from build123d import *

# Parameters (mm, degrees)
SKETCH1_R           = 5
SKETCH1_R_2         = 1.7
SKETCH1_R_3         = 2
SKETCH1_W           = 142.3736446
SKETCH1_H           = 35.551129401
SKETCH1_H_2         = 35.551129402
BOSS_EXTRUDE1_DEPTH = 2


with BuildPart() as part:
    # Sketch1 → Boss-Extrude1 (new body)
    with BuildSketch(Plane(origin=(0, 0, 0), x_dir=(1, 0, 0), z_dir=(0, 1, 0))):
        Polygon((67.730491212, 150.133829438), (82.230491212, 150.133829438), (85.730491212, 150.133829438), (85.730491212, 100.082700036), (85.730491212, 85.582700036), (85.730491212, 50.031570635), (85.730491212, 32.031570635), (67.730491212, 32.031570635), (62.730491212, 32.031570635), (62.730491212, 35.531570635), (-84.727026002, 35.531570635), (-99.227026002, 35.531570635), (-102.727026002, 35.531570635), (-102.727026002, 85.582700036), (-102.727026002, 92.832700036), (-102.727026002, 98.923608877), (-102.727026002, 100.082700036), (-102.727026002, 153.633829438), (-84.643153388, 153.633829438), (-79.643153388, 153.633829438), (-79.643153388, 153.432122466), (-79.643153388, 150.133829438), align=None)
        with Locations((-91.977026002, 142.883829438)):
            Circle(SKETCH1_R, mode=Mode.SUBTRACT)
        with Locations((74.980491212, 42.781570635)):
            Circle(SKETCH1_R, mode=Mode.SUBTRACT)
        with Locations((-86.427026002, 148.433829438)):
            Circle(SKETCH1_R_2, mode=Mode.SUBTRACT)
        with Locations((-97.527026002, 148.433829438)):
            Circle(SKETCH1_R_2, mode=Mode.SUBTRACT)
        with Locations((-86.427026002, 137.333829438)):
            Circle(SKETCH1_R_2, mode=Mode.SUBTRACT)
        with Locations((-97.527026002, 137.333829438)):
            Circle(SKETCH1_R_2, mode=Mode.SUBTRACT)
        with Locations((69.430491212, 48.331570635)):
            Circle(SKETCH1_R_2, mode=Mode.SUBTRACT)
        with Locations((80.530491212, 48.331570635)):
            Circle(SKETCH1_R_2, mode=Mode.SUBTRACT)
        with Locations((80.530491212, 37.231570635)):
            Circle(SKETCH1_R_2, mode=Mode.SUBTRACT)
        with Locations((69.430491212, 37.231570635)):
            Circle(SKETCH1_R_2, mode=Mode.SUBTRACT)
        with Locations((-54, 92.833829438)):
            Circle(SKETCH1_R_3, mode=Mode.SUBTRACT)
        with Locations((0, 92.833829438)):
            Circle(SKETCH1_R_3, mode=Mode.SUBTRACT)
        with Locations((54, 92.833829438)):
            Circle(SKETCH1_R_3, mode=Mode.SUBTRACT)
        with Locations((-8.456331088, 67.807135336)):
            Rectangle(SKETCH1_W, SKETCH1_H, mode=Mode.SUBTRACT)
        with Locations((-8.456331088, 117.858264737)):
            Rectangle(SKETCH1_W, SKETCH1_H_2, mode=Mode.SUBTRACT)
    extrude(amount=BOSS_EXTRUDE1_DEPTH)


solid = part.part
Here's how the part is built. I have some questions about the finished solid (model axes, mm). Round coordinates to 2 decimals unless told otherwise and drop trailing zeros. Loops run counter-clockwise (first coordinate to the right, second up) from the corner with the lowest first, then second, coordinate; pieces in that order, holes last. Notation, with made-up numbers: M 87.5,57 L 142.5,57 A15 cw 142.5,85 Z; hole C 19.5,27 d9. An arc over 180 degrees is marked long. Write each question's results on one line, items separated by ' | '. Start each with the question number.
(1) Will these pins go through, and if not, where does the flat tip stop? P1, Ø5.5, axis at x = 80.53, z = -37.23, coming from the -Y side; P2, Ø1, axis at x = -58, y = 1, coming from the +Z side.
(2) I want a section at C-C (x = -54). Please give me the cut outline in (y, z).
(3) Thinking about a two-plate mould opening in Z: for faces 1 (the flat face through (-7, 2, -94)), 2 (the cylindrical face through (-89.29, 0.99, -147.1)), which applies, pulls with the +Z half, pulls with the -Z half, needs draft (parallel to the pull), parting line crosses it, or undercut?
(4) I want a section at A-A (z = -59.5). Please give me the cut outline in (x, y), then the cut area to 3 significant figures.
(5) If I drill on probe 1 along Z at (x, y) = (-47, 1.2); probe 2 along X at (y, z) = (0.15, -114); probe 3 along X at (y, z) = (0.6, -91.5), over which ranges is the centre line in solid material (lowest first)? Write a range as from..to.
(6) I want a section at B-B (x = -12). Please give me the cut outline in (y, z).
(7) I want a section at D-D (y = 0.3). State how many separate pieces and enclosed holes the cut face has, then the cut area to 3 significant figures.
Solved:
1) P1: stops at y = 0 | P2: stops at z = -35.53
2) outline: M 0,-150.13 L 2,-150.13 L 2,-135.63 L 0,-135.63 Z; M 0,-100.08 L 2,-100.08 L 2,-94.83 L 0,-94.83 Z; M 0,-90.83 L 2,-90.83 L 2,-85.58 L 0,-85.58 Z; M 0,-50.03 L 2,-50.03 L 2,-35.53 L 0,-35.53 Z
3) face 1: needs draft | face 2: undercut
4) outline: M -102.73,0 L -79.64,0 L -79.64,2 L -102.73,2 Z; M 62.73,0 L 85.73,0 L 85.73,2 L 62.73,2 Z | area: 92.2 mm²
5) probe 1: z = -150.13..-135.63, -100.08..-85.58, -50.03..-35.53 | probe 2: x = -102.73..-79.64, 62.73..85.73 | probe 3: x = -102.73..-55.49, -52.51..-1.49, 1.49..52.51, 55.49..85.73
6) outline: M 0,-150.13 L 2,-150.13 L 2,-135.63 L 0,-135.63 Z; M 0,-100.08 L 2,-100.08 L 2,-85.58 L 0,-85.58 Z; M 0,-50.03 L 2,-50.03 L 2,-35.53 L 0,-35.53 Z
7) separate pieces: 1 | enclosed holes: 15 | area: 11,400 mm²
